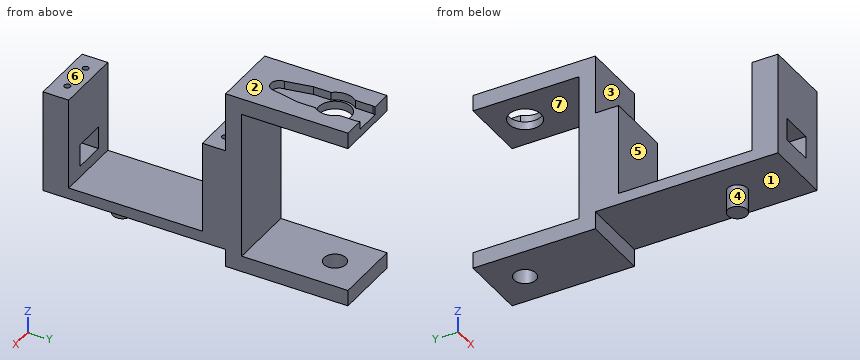
from build123d import *

# Parameters (mm, degrees)
CYLINDER030_R     = 3.4
CYLINDER030_DEPTH = 44
CYLINDER029_R     = 5
CYLINDER029_DEPTH = 9
PAD010_DEPTH      = 5
PAD009_DEPTH      = 21
CYLINDER034_R     = 0.95
CYLINDER034_DEPTH = 10
CYLINDER035_R     = 0.95
CYLINDER035_DEPTH = 10
CYLINDER032_R     = 0.95
CYLINDER032_DEPTH = 10
CYLINDER033_R     = 0.95
CYLINDER033_DEPTH = 10
BOX006_W          = 10
BOX006_H          = 10
BOX006_DEPTH      = 7
PAD011_DEPTH      = 21
CYLINDER031_R     = 3
CYLINDER031_DEPTH = 10


with BuildPart() as cylinder030:
    # Cylinder030 → Cylinder030 (new body)
    with BuildSketch(Plane(origin=(10.5, -10.1, -9), x_dir=(1, 0, 0), z_dir=(0, 0, 1))):
        Circle(CYLINDER030_R)
    extrude(amount=CYLINDER030_DEPTH)


with BuildPart() as cylinder029:
    # Cylinder029 → Cylinder029 (new body)
    with BuildSketch(Plane(origin=(10.5, -10.1, 45), x_dir=(1, 0, 0), z_dir=(0, 0, 1))):
        Circle(CYLINDER029_R)
    extrude(amount=CYLINDER029_DEPTH)


with BuildPart() as fusion024:
    # Sketch010 → Pad010 (new body)
    with BuildSketch(Plane.XY):
        with BuildLine():
            Line((-4.25, 3.75), (-4.25, 9.25))
            Line((-4.25, 9.25), (-2.65, 17.292388))
            ThreePointArc((2.65, 17.292388), (0, 20), (-2.65, 17.292388))
            Line((2.65, 17.292388), (4.25, 9.25))
            Line((4.25, 3.75), (4.25, 9.25))
            ThreePointArc((4.25, -3.75), (5.657274, 0), (4.25, 3.75))
            Line((4.25, -3.75), (4.25, -9.25))
            Line((2.65, -17.292388), (4.25, -9.25))
            ThreePointArc((-2.65, -17.292388), (0, -20), (2.65, -17.292388))
            Line((-4.25, -9.25), (-2.65, -17.292388))
            Line((-4.25, -3.75), (-4.25, -9.25))
            ThreePointArc((-4.25, 3.75), (-5.657274, 0), (-4.25, -3.75))
        make_face()
    extrude(amount=PAD010_DEPTH)


with BuildPart() as fusion024_1:
    # Body010 placement: moved
    add(fusion024.part.moved(Location((10.5, -10, 48))))

    # Fusion024: union Cylinder029
    add(cylinder029.part)


with BuildPart() as obj1:
    # Sketch009 → Pad009 (new body)
    with BuildSketch(Plane.YZ):
        Polygon((-33, -0.5), (0, -0.5), (0, -5.5), (-38, -5.5), (-38, 50.5), (0, 50.5), (0, 45.5), (-33, 45.5), align=None)
    extrude(amount=PAD009_DEPTH)

    # Cut014: cut Fusion024
    add(fusion024_1.part, mode=Mode.SUBTRACT)

    # Cut015: cut Cylinder030
    add(cylinder030.part, mode=Mode.SUBTRACT)


with BuildPart() as cylinder034:
    # Cylinder034 → Cylinder034 (new body)
    with BuildSketch(Plane(origin=(9.9, 0, 0), x_dir=(1, 0, 0), z_dir=(0, 0, 1))):
        Circle(CYLINDER034_R)
    extrude(amount=CYLINDER034_DEPTH)


with BuildPart() as tornillos013:
    # Cylinder035 → Cylinder035 (new body)
    with BuildSketch(Plane.XY):
        Circle(CYLINDER035_R)
    extrude(amount=CYLINDER035_DEPTH)

    # Fusion026: union Cylinder034
    add(cylinder034.part)


with BuildPart() as tornillos013_1:
    # Fusion026 placement: moved
    add(tornillos013.part.moved(Location((5, -24.5, 22))))


with BuildPart() as cylinder032:
    # Cylinder032 → Cylinder032 (new body)
    with BuildSketch(Plane(origin=(9.9, 0, 0), x_dir=(1, 0, 0), z_dir=(0, 0, 1))):
        Circle(CYLINDER032_R)
    extrude(amount=CYLINDER032_DEPTH)


with BuildPart() as fusion027:
    # Cylinder033 → Cylinder033 (new body)
    with BuildSketch(Plane.XY):
        Circle(CYLINDER033_R)
    extrude(amount=CYLINDER033_DEPTH)

    # Fusion025: union Cylinder032
    add(cylinder032.part)


with BuildPart() as fusion027_1:
    # Fusion025 placement: moved
    add(fusion027.part.moved(Location((5, 24.5, 22))))

    # Fusion027: union Tornillos013
    add(tornillos013_1.part)


with BuildPart() as fusion027_2:
    # Fusion027 placement: moved
    add(fusion027_1.part.moved(Location((0.4, 0, 0))))


with BuildPart() as cube006:
    # Box006 → Box006 (new body)
    with BuildSketch(Plane(origin=(5, -29, 7), x_dir=(1, 0, 0), z_dir=(0, 0, 1))):
        with Locations((5, 5)):
            Rectangle(BOX006_W, BOX006_H)
    extrude(amount=BOX006_DEPTH)


with BuildPart() as holder007:
    # Sketch011 → Pad011 (new body)
    with BuildSketch(Plane.YZ):
        Polygon((-28.75, 32), (-28.75, 0), (28.75, 0), (28.75, 32), (20.75, 32), (20.75, 3.5), (-20.75, 3.5), (-20.75, 32), align=None)
    extrude(amount=PAD011_DEPTH)

    # Cut016: cut Cube006
    add(cube006.part, mode=Mode.SUBTRACT)

    # Cut017: cut Fusion027
    add(fusion027_2.part, mode=Mode.SUBTRACT)


with BuildPart() as fusion029:
    # Cylinder031 → Cylinder031 (new body)
    with BuildSketch(Plane(origin=(10.5, -10.1, -7), x_dir=(1, 0, 0), z_dir=(0, 0, 1))):
        Circle(CYLINDER031_R)
    extrude(amount=CYLINDER031_DEPTH)

    # Fusion028: union Holder007
    add(holder007.part)


with BuildPart() as fusion029_1:
    # Fusion028 placement: moved
    add(fusion029.part.moved(Location((0, -66, 0))))

    # Fusion029: union obj1
    add(obj1.part)


solid = fusion029_1.part
The model under review builds one solid part; all positions refer to its coordinate system, in mm. Face numbers are marked on the shaded views. A direction names the side the tool comes from. Round coordinates to 2 decimals unless told otherwise and drop trailing zeros. Loops run counter-clockwise (first coordinate to the right, second up) from the corner with the lowest first, then second, coordinate; pieces in that order, holes last. Notation, with made-up numbers: (56.5, 15.25) -> (77.5, 15.25) arc R11 cw to (77.5, 24.25) -> close; hole circle Ø8 at (33.25, 30.25). An arc over 180 degrees is marked (long way). Return JSON: item names as keys, results as strings.
(1) For line 1 (Y direction, x = 5.4, z = 25.75); line 2 (Y direction, x = 10.5, z = -2.5); line 3 (Y direction, x = 18, z = 21), list the stretches that pass through material, from the lowest coordinate up.
Solved:
{"line 1": "-94.75 to -91.45, -89.55 to -86.75, -45.25 to -42.45, -40.55 to -33", "line 2": "-79.1 to -73.1, -38 to -13.5, -6.7 to 0", "line 3": "-94.75 to -86.75, -45.25 to -33"}
(2) Add section A-A on x = 10.5. State how many separate pieces and enclosed holes the cut face has, plus the area to 3 significant figures.
Solved:
{"separate pieces": "4", "enclosed holes": "0", "area": "1,100 mm2"}
(3) Add section B-B on z = 25. Write out the cut boundary in (x, y), plus the area to 3 significant figures.
Solved:
{"outline": "(0, -94.75) -> (21, -94.75) -> (21, -86.75) -> (0, -86.75) -> close; (0, -45.25) -> (21, -45.25) -> (21, -33) -> (0, -33) -> close; hole circle Ø1.9 at (5.4, -90.5); hole circle Ø1.9 at (5.4, -41.5); hole circle Ø1.9 at (15.3, -90.5); hole circle Ø1.9 at (15.3, -41.5)", "area": "414 mm2"}
(4) For the marked faces 4, 5, 6 and 7, list the 3-axis set-ups (+Z, -Z, +X, -X, +Y, -Y) from which the entire face can be reached by the end or side of a thin tool; tool diameter is ignored.
Solved:
{"face 4": "-Z", "face 5": "+Z, +X, -X", "face 6": "+Z, +X, -X, -Y", "face 7": "+X, -X, +Y"}
(5) Add section C-C on z = -2.5. Write out the cut boundary in (x, y).
Solved:
{"outline": "(0, -38) -> (21, -38) -> (21, 0) -> (0, 0) -> close; circle Ø6 at (10.5, -76.1); hole circle Ø6.8 at (10.5, -10.1)"}
(6) The part is to be moulded in two halves that separate along Y. For the marked faces 1, 2 and 3, say which applies: released by +Y, released by -Y, zero draft, split by the parting line, or undercut.
Solved:
{"face 1": "undercut", "face 2": "zero draft", "face 3": "released by -Y"}
(7) Add section D-D on y = -41.5. Write out the cut boundary in (x, z).
Solved:
{"outline": "(0, 0) -> (21, 0) -> (21, 32) -> (16.25, 32) -> (16.25, 22) -> (14.35, 22) -> (14.35, 32) -> (6.35, 32) -> (6.35, 22) -> (4.45, 22) -> (4.45, 32) -> (0, 32) -> close"}
(8) For pin 1 (5.5 mm diameter, centred on x = 11.5, z = 39, fed in from -Y); pin 2 (10 mm diameter, centred on x = 17.5, y = -60.5, fed in from -Z); pin 3 (6.5 mm diameter, centred on x = 12.5, y = -92, fed in from +Z), all flat-tipped, find the tip position at first contact; note any pin that passes through.
Solved:
{"pin 1": "y = -38", "pin 2": "z = 0", "pin 3": "z = 32"}
